Input: part model. Units: mm. Frame: model coordinates. Coordinates: 2 decimals unless noted, no trailing zeros. Write each loop counter-clockwise with the first axis right and the second up, starting at its lowest first coordinate (ties: lowest second). Pieces come first, ordered by that corner, then holes.
1) Section query B-B (z = -28). Output: boundary loops of the cut face in (x, y), then the cut area to 3 significant figures.
2) Section query C-C (y = 6). Output: boundary loops of the cut face in (x, z), then the cut area to 3 significant figures.
3) Section query A-A (x = 0). Output: boundary loops of the cut face in (y, z).
4) Pin query (flat end, axial travel): pin 1 Ø2 at (x, y) = (4.5, 3.5) entering from +Z. Return the tip coordinate at first contact, or that it passes through.
5) Line query: L1, parallel to Z at x = -4, y = 6; L2, parallel to Z at x = 16.5, y = 7; L3, parallel to X at y = 5.5, z = 27. Output: solid intervals per line, ascending.
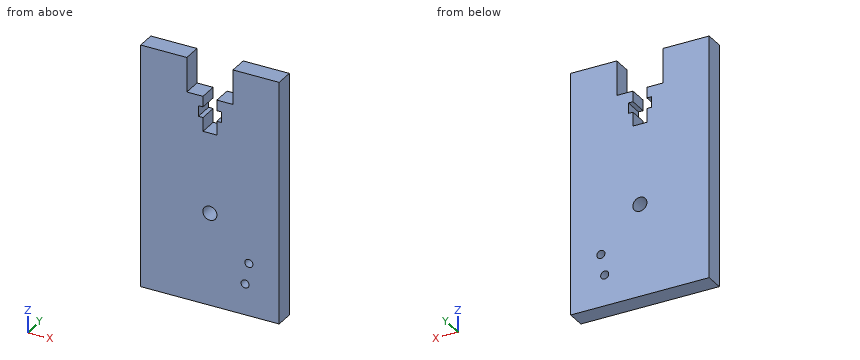
from build123d import *

# Parameters (mm, degrees)
SKETCH1_R           = 3.05
SKETCH1_R_2         = 1.75
BOSS_EXTRUDE1_DEPTH = 8


with BuildPart() as part:
    # Sketch1 → Boss-Extrude1 (new body)
    with BuildSketch(Plane(origin=(0, 0, 0), x_dir=(1, 0, 0), z_dir=(0, 1, 0))):
        Polygon((-10, -37), (-10, -22), (-3, -22), (-3, -17.4), (-5, -17.4), (-5, -12.8), (-3, -12.8), (-3, -6.8), (3, -6.8), (3, -12.8), (5, -12.8), (5, -17.4), (3, -17.4), (3, -22), (10, -22), (10, -37), (30, -37), (30, 38), (30, 58), (30, 68), (-30, 68), (-30, 58), (-30, 38), (-30, -37), align=None)
        with Locations(Location((0, 28, 0), (0, 0, 270))):
            Circle(SKETCH1_R, mode=Mode.SUBTRACT)
        with Locations(Location((16.89444432, 45.232293128, 0), (0, 0, 270))):
            Circle(SKETCH1_R_2, mode=Mode.SUBTRACT)
        with Locations(Location((15.244786632, 54.587966781, 0), (0, 0, 90))):
            Circle(SKETCH1_R_2, mode=Mode.SUBTRACT)
    extrude(amount=BOSS_EXTRUDE1_DEPTH)


solid = part.part
Answer:
1. outline: (-30, 0) - (-3.05, 0) - (-3.05, 8) - (-30, 8) - close; (3.05, 0) - (30, 0) - (30, 8) - (3.05, 8) - close
1. area: 431 mm2
2. outline: (-30, -68) - (30, -68) - (30, 37) - (10, 37) - (10, 22) - (3, 22) - (3, 17.4) - (5, 17.4) - (5, 12.8) - (3, 12.8) - (3, 6.8) - (-3, 6.8) - (-3, 12.8) - (-5, 12.8) - (-5, 17.4) - (-3, 17.4) - (-3, 22) - (-10, 22) - (-10, 37) - (-30, 37) - close; hole circle Ø6.1 at (0, -28); hole circle Ø3.5 at (15.24, -54.59); hole circle Ø3.5 at (16.89, -45.23)
2. area: 5,840 mm2
3. outline: (0, -68) - (8, -68) - (8, -31.05) - (0, -31.05) - close; (0, -24.95) - (8, -24.95) - (8, 6.8) - (0, 6.8) - close
4. pin 1: stops at z = 22
5. L1: z = -68 to 12.8, 17.4 to 22
5. L2: z = -68 to -55.81, -53.37 to -46.94, -43.53 to 37
5. L3: x = -30 to -10, 10 to 30
